Can you work these out from the drawing? Everything is in mm from the part's minimum corner. Give positions to 0.01 mm unless a question says otherwise; leave off trailing zeros. Order: outer loops, then holes, each group sorted by start corner. A loop starts at its lowest first (then second) coordinate and runs counter-clockwise, first axis right, second up. Notation, with made-up numbers: (69, -22) -> (91, -22) arc R16 cw to (91, 9) -> close; hole circle Ø9 at (-6.5, 58). An arc over 180 degrees is marked (long way). One line per item, written item: value.
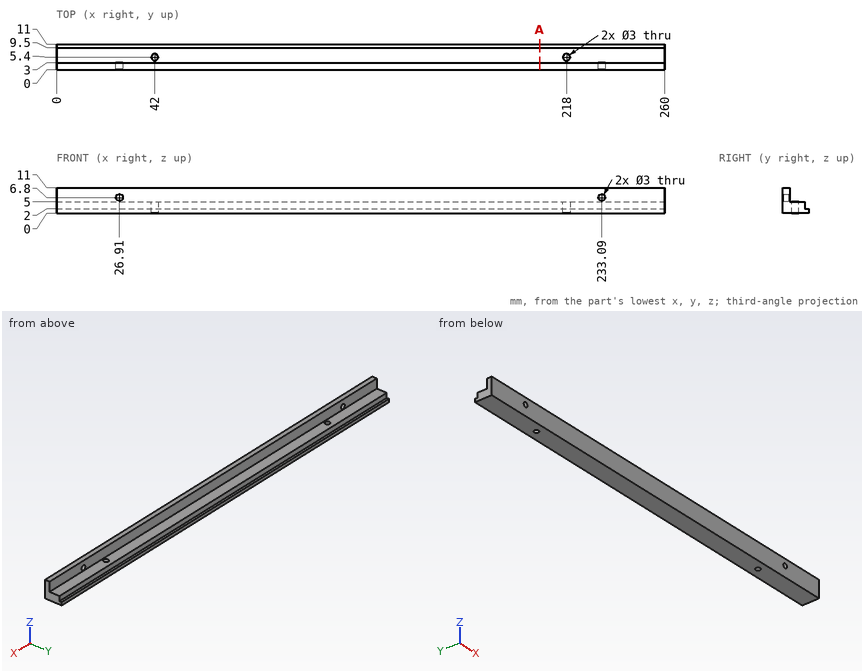
1) For P1, Ø5, axis at x = 26.91, z = 6.8, coming from the -Y side; P2, Ø1.6, axis at x = 86.5, y = 10, coming from the +Z side; P3, Ø4, axis at x = 96.5, z = 7.5, coming from the +Y side; P4, Ø5, axis at x = 104.5, z = 7, coming from the +Y side, each with a flat end and sliding along its axis, tell me the tip position at first contact or that it passes through.
Answer below:
P1: stops at y = 0
P2: stops at z = 5
P3: stops at y = 3
P4: stops at y = 9.5
2) Suppose I cut it at A-A, the plane x = 206.5. Write out the boundary of the cut face in (y, z), then the cut area to 3 significant figures.
Answer below:
outline: (0, 0) -> (11, 0) -> (11, 2) -> (9.5, 2) -> (9.5, 5) -> (3, 5) -> (3, 11) -> (0, 11) -> close
area: 68.5 mm2
3) If I drill on line 1 along X through (y, z) = (2.35, 6.8); line 2 along X through (y, z) = (4.5, 3.75); line 3 along Y through (x, z) = (42, 2.75), over which ranges is the centre line in solid material (lowest first)?
Answer below:
line 1: x = 0 to 25.41, 28.41 to 231.59, 234.59 to 260
line 2: x = 0 to 40.8, 43.2 to 216.8, 219.2 to 260
line 3: y = 0 to 3.9, 6.9 to 9.5
